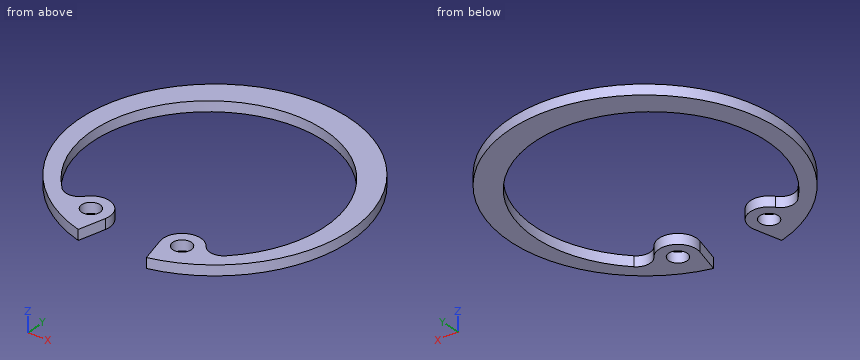
from build123d import *

# Parameters (mm, degrees)
BODYSKE_R  = 1
BODY_DEPTH = 1.1


with BuildPart() as part:
    # BodySke → Body (new body)
    with BuildSketch(Plane.XY):
        with BuildLine():
            Line((3.698325427, -14.227170802), (2.961893262, -11.394173437))
            ThreePointArc((2.961893262, -11.394173437), (4.055312562, -9.032003244), (6.584655155, -9.646690019))
            ThreePointArc((6.584655155, -9.646690019), (7.702025194, -10.256332456), (8.895921915, -9.814981887))
            ThreePointArc((8.895921915, -9.814981887), (0, 11.8), (-8.895921915, -9.814981887))
            ThreePointArc((-8.895921915, -9.814981887), (-7.702025194, -10.256332456), (-6.584655155, -9.646690019))
            ThreePointArc((-6.584655155, -9.646690019), (-4.055312562, -9.032003244), (-2.961893262, -11.394173437))
            Line((-2.961893262, -11.394173437), (-3.698325427, -14.227170802))
            ThreePointArc((-3.698325427, -14.227170802), (0, 14.7), (3.698325427, -14.227170802))
        make_face()
        with Locations((4.945954497, -10.878420571)):
            Circle(BODYSKE_R, mode=Mode.SUBTRACT)
        with Locations((-4.945954497, -10.878420571)):
            Circle(BODYSKE_R, mode=Mode.SUBTRACT)
    extrude(amount=-BODY_DEPTH)


solid = part.part
Verification items for the finished model (mm, model axes). Give positions to 0.01 mm unless a question says otherwise; leave off trailing zeros. Order: outer loops, then holes, each group sorted by start corner. A loop starts at its lowest first (then second) coordinate and runs counter-clockwise, first axis right, second up. Notation, with made-up numbers: M 72.25,70.25 L 92.25,70.25 A16 ccw 92.25,78.25 Z; hole C -13.75,85 d11. An arc over 180 degrees is marked long. Answer as a JSON object with one key per item and string values. Group by question number.
1) Cross-section at B-B (z = -0.3). Give the number of separate pieces and of enclosed holes in the cut face, then the cut area to 3 significant figures.
2) Cross-section at A-A (y = -8.25). Enter the section's corners in (x, z).
3) Cross-section at D-D (x = 0). Enter the section's corners in (y, z).
4) Cross-section at C-C (y = 1). Enter the section's corners in (x, z), then the cut area to 3 significant figures.
5) Scan lines: line 1 along X through (y, z) = (-9, -0.55); line 2 along X through (y, z) = (-11.5, -0.6); line 3 along Y through (x, z) = (10.5, -0.8). Record each from-to range of solid material in increasing order. Write a range as [from, to].
Result sheet:
{
 "1": {"separate pieces": "1", "enclosed holes": "2", "area": "189 mm2"},
 "2": {"outline": "M -12.17,-1.1 L -10.24,-1.1 L -10.24,0 L -12.17,0 Z; M 10.24,-1.1 L 12.17,-1.1 L 12.17,0 L 10.24,0 Z"},
 "3": {"outline": "M 11.8,-1.1 L 14.7,-1.1 L 14.7,0 L 11.8,0 Z"},
 "4": {"outline": "M -14.67,-1.1 L -12.5,-1.1 L -12.5,0 L -14.67,0 Z; M 12.5,-1.1 L 14.67,-1.1 L 14.67,0 L 12.5,0 Z", "area": "4.76 mm2"},
 "5": {"line 1": "x = [-11.62, -9.65], [-5.77, -4.12], [4.12, 5.77], [9.65, 11.62]", "line 2": "x = [-9.16, -5.73], [-4.16, -2.99], [2.99, 4.16], [5.73, 9.16]", "line 3": "y = [-10.29, -7.87], [6.2, 10.29]"}
}
